Work out the finished part from the listing and answer in its coordinate system (mm). Face numbers are marked on the shaded views. Give positions to 0.01 mm unless a question says otherwise; leave off trailing zeros. Use a Markdown table: item, result.
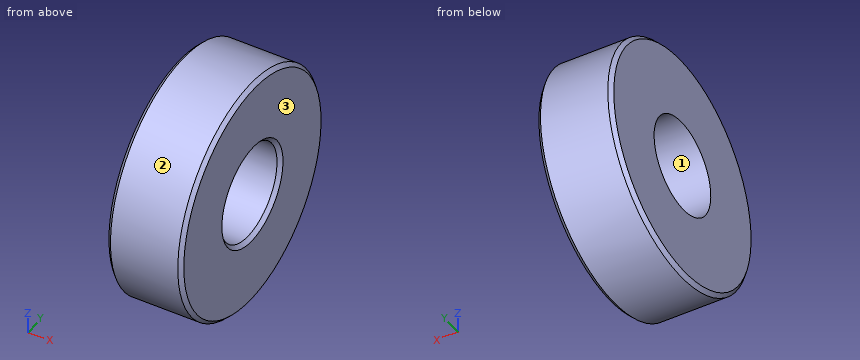
```python
from build123d import *

# Parameters (mm, degrees)
SKETCH1_R           = 7.9375
SKETCH1_R_2         = 3.175
BOSS_EXTRUDE1_DEPTH = 2.489
CHAMFER1_SIZE       = 0.25


with BuildPart() as part:
    # Sketch1 → Boss-Extrude1 (new, symmetric)
    with BuildSketch(Plane(origin=(0, 0, 0), x_dir=(0, 0, -1), z_dir=(1, 0, 0))):
        Circle(SKETCH1_R)
        Circle(SKETCH1_R_2, mode=Mode.SUBTRACT)
    extrude(amount=BOSS_EXTRUDE1_DEPTH, both=True)

    # Chamfer1
    chamfer1_edges = [part.edges().sort_by_distance(p)[0] for p in [
        (-2.489, 0, 7.9375),
        (2.489, 0, 7.9375),
        (2.489, 0, 3.175),
    ]]
    chamfer(chamfer1_edges, length=CHAMFER1_SIZE)


solid = part.part
```
(1) The mould has two halves that part along Y. Classify the marked faces 1, 2 and 3: released by +Y, released by -Y, zero draft, split by the parting line, or undercut.
Entries:
| item | result |
|---|---|
| face 1 | undercut |
| face 2 | split by the parting line |
| face 3 | zero draft |
(2) Given P1, Ø1, axis at x = 0, z = -5.5, coming from the -Y side, flat-ended and moving along its own axis, determine where the tip first touches the part or whether it passes through.
Entries:
| item | result |
|---|---|
| P1 | stops at y = -6.16 |
(3) Consider probe 1 along Y at (x, z) = (-1.1, 0) (1 decimal); probe 2 along Y at (x, z) = (-0.9, -2); probe 3 along Z at (x, y) = (1, 0.5). Determine where each line is inside the solid, lowest interval first. Write a range as [from, to].
Entries:
| item | result |
|---|---|
| probe 1 | y = [-7.9, -3.2], [3.2, 7.9] |
| probe 2 | y = [-7.68, -2.47], [2.47, 7.68] |
| probe 3 | z = [-7.92, -3.14], [3.14, 7.92] |
